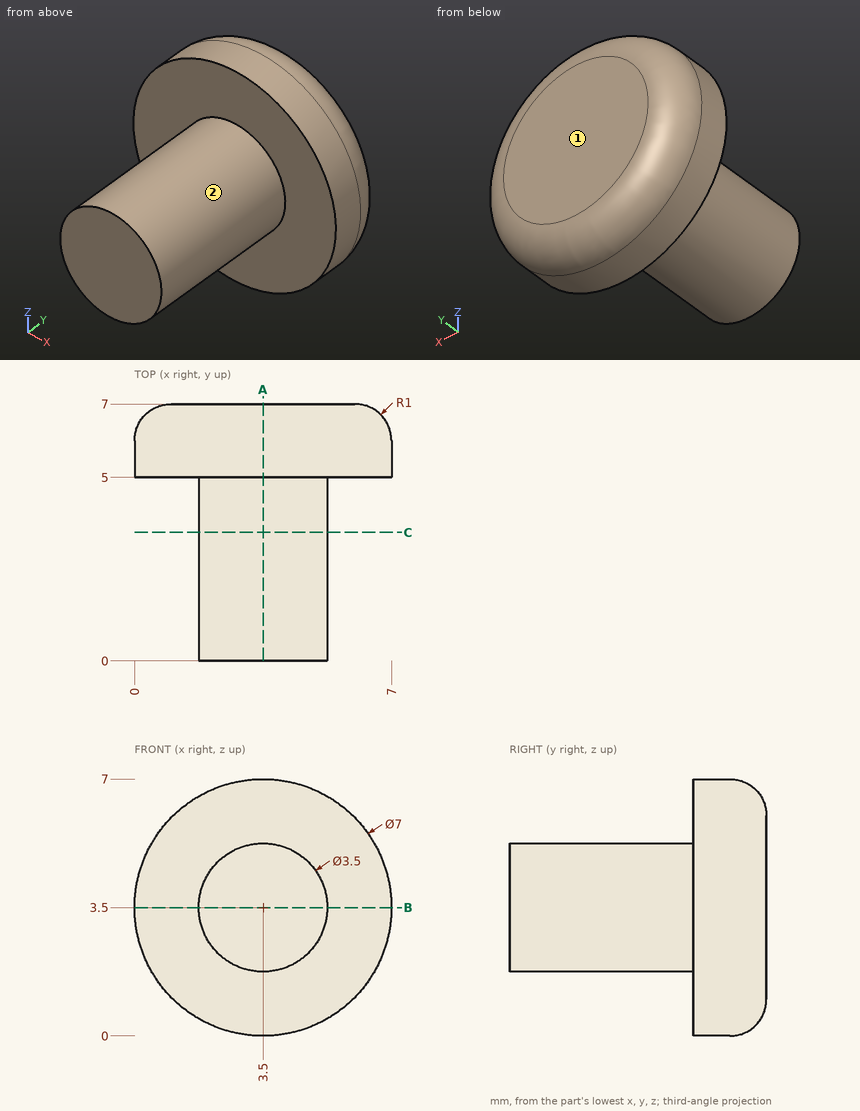
Geometry check sheet. Reference: drawing and pictorial views, mm from the part's lowest x, y, z. A direction names the side the tool comes from. Give positions to 0.01 mm unless a question says otherwise; leave off trailing zeros. Order: outer loops, then holes, each group sorted by start corner. A loop starts at its lowest first (then second) coordinate and runs counter-clockwise, first axis right, second up. Notation, with made-up numbers: M 23.25,24 L 63.25,24 A20 ccw 63.25,59 Z; hole C -8,31 d9. An arc over 180 degrees is marked long. Answer in a Markdown table with one row per item. Add a question column.
Q1. Access from +Z, -Z, +X, -X, +Y, -Y to the whole of each face (thin tool, end or side, straight path). Record for the marked faces 1 and 2.
Q2. Sectioned sample at C-C, the plane y = 3.5. Record the boundary of the cut face in (x, z).
Q3. Sectioned sample at B-B, the plane z = 3.5. Record the boundary of the cut face in (x, y), and give its area (3 significant figures).
Q4. Thickness scan on L1, parallel to Y at x = 3, z = 5.5; L2, parallel to X at y = 1.5, z = 3.5; L3, parallel to X at y = 4.25, z = 2. Record the ranges inside material, lowest first.
Q5. Sectioned sample at A-A, the plane x = 3.5. Record the boundary of the cut face in (y, z).
Q6. Gauge pin test, flat end, axial feed: pin 1 Ø4 at (y, z) = (1.5, 3) entering from +X. Record the tip position at first contact, or that the pin passes through.
Verdict:
| question | item | result |
|---|---|---|
| 1 | face 1 | +Z, -Z, +X, -X, +Y |
| 1 | face 2 | -Y |
| 2 | outline | C 3.5,3.5 d3.5 |
| 3 | outline | M 0,5 L 1.75,5 L 1.75,0 L 5.25,0 L 5.25,5 L 7,5 L 7,6 A1 ccw 6,7 L 1,7 A1 ccw 0,6 Z |
| 3 | area | 31.1 mm² |
| 4 | L1 | 5 to 7 |
| 4 | L2 | 1.75 to 5.25 |
| 4 | L3 | 2.6 to 4.4 |
| 5 | outline | M 0,1.75 L 5,1.75 L 5,0 L 6,0 A1 ccw 7,1 L 7,6 A1 ccw 6,7 L 5,7 L 5,5.25 L 0,5.25 Z |
| 6 | pin 1 | x = 5.25 |
